Verification items for the finished model (mm, model axes). Round coordinates to 2 decimals unless told otherwise and drop trailing zeros. Write each loop counter-clockwise with the first axis right and the second up, starting at its lowest first coordinate (ties: lowest second). Pieces come first, ordered by that corner, then holes. Notation, with made-up numbers: (22, 75.25) - (41, 75.25) arc R10 ccw to (41, 92.25) - close; hole circle Ø1 at (34.5, 80). An arc over 180 degrees is marked (long way). Answer as a JSON object with one key per item and string values.
```python
from build123d import *

# Parameters (mm, degrees)
MODEL_R                 = 36
MODEL_R_2               = 4.5
MODEL_R_3               = 1.5
SALIENTE_EXTRUIR1_DEPTH = 3


with BuildPart() as part:
    # Model → Saliente-Extruir1 (new body)
    with BuildSketch(Plane.XY):
        with Locations((225.25945398, 284.786767066)):
            Circle(MODEL_R)
        with Locations((207.25945398, 302.786767066)):
            Circle(MODEL_R_2, mode=Mode.SUBTRACT)
        with Locations((207.25945398, 266.786767066)):
            Circle(MODEL_R_2, mode=Mode.SUBTRACT)
        with Locations((243.25945398, 266.786767066)):
            Circle(MODEL_R_2, mode=Mode.SUBTRACT)
        with Locations((243.25945398, 302.786767066)):
            Circle(MODEL_R_2, mode=Mode.SUBTRACT)
        with Locations((225.25945398, 284.786767066)):
            Circle(MODEL_R_3, mode=Mode.SUBTRACT)
        with Locations((225.25945398, 275.786767066)):
            Circle(MODEL_R_3, mode=Mode.SUBTRACT)
        with Locations((225.25945398, 293.786767066)):
            Circle(MODEL_R_3, mode=Mode.SUBTRACT)
        with Locations((234.25945398, 284.786767066)):
            Circle(MODEL_R_3, mode=Mode.SUBTRACT)
        with Locations((216.25945398, 284.786767066)):
            Circle(MODEL_R_3, mode=Mode.SUBTRACT)
        with Locations((243.25945398, 284.786767066)):
            Circle(MODEL_R_3, mode=Mode.SUBTRACT)
        with Locations((252.25945398, 284.786767066)):
            Circle(MODEL_R_3, mode=Mode.SUBTRACT)
        with Locations((198.25945398, 284.786767066)):
            Circle(MODEL_R_3, mode=Mode.SUBTRACT)
        with Locations((207.25945398, 284.786767066)):
            Circle(MODEL_R_3, mode=Mode.SUBTRACT)
        with Locations((225.25945398, 302.786767066)):
            Circle(MODEL_R_3, mode=Mode.SUBTRACT)
        with Locations((225.25945398, 311.786767066)):
            Circle(MODEL_R_3, mode=Mode.SUBTRACT)
        with Locations((225.25945398, 266.786767066)):
            Circle(MODEL_R_3, mode=Mode.SUBTRACT)
        with Locations((225.25945398, 257.786767066)):
            Circle(MODEL_R_3, mode=Mode.SUBTRACT)
        with Locations((216.25945398, 275.786767066)):
            Circle(MODEL_R_3, mode=Mode.SUBTRACT)
        with Locations((234.25945398, 293.786767066)):
            Circle(MODEL_R_3, mode=Mode.SUBTRACT)
        with Locations((234.25945398, 275.786767066)):
            Circle(MODEL_R_3, mode=Mode.SUBTRACT)
        with Locations((216.25945398, 293.786767066)):
            Circle(MODEL_R_3, mode=Mode.SUBTRACT)
    extrude(amount=SALIENTE_EXTRUIR1_DEPTH)


solid = part.part
```
1. Cross-section at B-B (x = 255). Record the boundary of the cut face in (y, z), plus the area to 3 significant figures.
Completed:
{"outline": "(264.5, 0) - (305.07, 0) - (305.07, 3) - (264.5, 3) - close", "area": "122 mm^2"}
2. Go/stop test with a flat-tipped pin: pin 1 (1 mm diameter, centred on y = 295, z = 0.5, fed in from -X). Record where the tip stops, or that it passes through.
Completed:
{"pin 1": "stops at x = 190.59"}
3. Mould release check, pull along Y, two halves, no side actions. Record for faces 1 (the face through (220.57, 320.48, 1.48)), 2 (the face through (233, 277, 3)), 3 (the face through (225.064, 304.274, 1.479)): released by +Y, released by -Y, zero draft, split by the parting line, or undercut.
Completed:
{"face 1": "split by the parting line", "face 2": "zero draft", "face 3": "undercut"}
4. Material ranges on probe 1 along X at (y, z) = (300, 1.1); probe 2 along Y at (x, z) = (215, 2.6); probe 3 along X at (y, z) = (275.5, 0.85), recorded low to high. Write a range as from..to.
Completed:
{"probe 1": "x = 192.63..203.73, 210.79..239.73, 246.79..257.89", "probe 2": "y = 250.28..274.97, 276.6..283.97, 285.6..292.97, 294.6..319.29", "probe 3": "x = 190.48..214.79, 217.73..223.79, 226.73..232.79, 235.73..260.04"}
5. Cross-section at A-A (z = 1.55). Count the separate pieces of the cut face and the enclosed holes in it, plus the area to 3 significant figures.
Completed:
{"separate pieces": "1", "enclosed holes": "21", "area": "3,700 mm^2"}
6. Cross-section at C-C (y = 253). Record the boundary of the cut face in (x, z), plus the area to 3 significant figures.
Completed:
{"outline": "(208.36, 0) - (242.16, 0) - (242.16, 3) - (208.36, 3) - close", "area": "101 mm^2"}
